Autodesk Inventor part; units mm, degrees
ref_plane "YZ Plane" through (0, 0, 0) normal (1, 0, 0) x (0, 1, 0)
ref_plane "XZ Plane" through (0, 0, 0) normal (0, 1, 0) x (-1, 0, 0)
ref_plane "XY Plane" through (0, 0, 0) normal (0, 0, 1) x (1, 0, 0)
sketch "Sketch1" plane through (0, 0, 0) normal (0, 1, 0) x (-1, 0, 0)
  line L0 (0, 0) -> (-10.25, 0)
  line L1 (-10.25, 0) -> (-10.25, -60)
  line L2 (-14.25, 4) -> (0, 4)
  line L3 (0, 4) -> (0, 0)
  line L4 (-10.25, -60) -> (-30.25, -60)
  line L5 (-30.25, -60) -> (-30.25, -56)
  line L6 (-30.25, -56) -> (-14.25, -56)
  line L7 (-14.25, -56) -> (-14.25, 4)
  dimension "d0" = 10.25
  dimension "d1" = 60
  dimension "d3" = 4
  dimension "d4" = 20
  dimension "d5" = 4
  dimension "d6" = 4
extrude "Extrusion1" add sketch "Sketch1" along normal blind 15
sketch "Sketch2" plane through (14.25, 0, -56) normal (0, 0, 1) x (1, 0, 0)
  line L0 (0, 15) -> (16, 0) construction
  line L1 (0, 0) -> (16, 15) construction
  point P0 (-14.25, 0)
  point P1 (8, 7.5)
hole "Hole1" at (22.25, 7.5, -56) direction (0, 0, -1) diameter 3.5 depth 8 tip angle 118
mirror "Mirror1" about plane through (0, 0, 0) normal (-1, 0, 0)
properties part number "clip" material "ABS Plastic"
Input: part model. Units: mm. Frame: model coordinates. A direction names the side the tool comes from. Round coordinates to 2 decimals unless told otherwise and drop trailing zeros. Loops run counter-clockwise (first coordinate to the right, second up) from the corner with the lowest first, then second, coordinate; pieces in that order, holes last. Notation, with made-up numbers: (35.25, 44.25) -> (69.25, 44.25) arc R8 ccw to (69.25, 54.25) -> close; hole circle Ø1 at (48.5, 26.25). An arc over 180 degrees is marked (long way). Write each question's results on one line, items separated by ' | '.
1. Ray query, line 1 (X direction, y = 7.5, z = -59.1); line 2 (X direction, y = 13, z = -21); line 3 (Y direction, x = -22, z = -58). Return the intervals inside material, ascending. Write a range as from..to.
Geometry results:
line 1: -30.25..-24, -20.5..-10.25, 10.25..20.5, 24..30.25 | line 2: -14.25..-10.25, 10.25..14.25 | line 3: 0..5.77, 9.23..15
2. Section B-B (y = 7.5). Return loops of the section in (x, z), and give its area (3 significant figures).
Geometry results:
outline: (-30.25, -60) -> (-24, -60) -> (-24, -56) -> (-30.25, -56) -> close; (-20.5, -60) -> (-10.25, -60) -> (-10.25, 0) -> (10.25, 0) -> (10.25, -60) -> (20.5, -60) -> (20.5, -56) -> (14.25, -56) -> (14.25, 4) -> (-14.25, 4) -> (-14.25, -56) -> (-20.5, -56) -> close; (24, -60) -> (30.25, -60) -> (30.25, -56) -> (24, -56) -> close | area: 694 mm2
3. First-contact query: P1, Ø5, axis at y = 11, z = -36.5, coming from the +X side; P2, Ø8, axis at x = -21.5, z = -44.5, coming from the -Y side; P3, Ø4.5, axis at y = 4, z = -18, coming from the -X side; P4, Ø5.5, axis at x = 22.25, y = 7.5, coming from the +Z side. Flat tips, straight axial feed; report the tip coordinate or a pass-through.
Geometry results:
P1: x = 14.25 | P2: through | P3: x = -14.25 | P4: z = -56
4. Section D-D (y = 12.5). Return loops of the section in (x, z), and give its area (3 significant figures).
Geometry results:
outline: (-30.25, -60) -> (-10.25, -60) -> (-10.25, 0) -> (10.25, 0) -> (10.25, -60) -> (30.25, -60) -> (30.25, -56) -> (14.25, -56) -> (14.25, 4) -> (-14.25, 4) -> (-14.25, -56) -> (-30.25, -56) -> close | area: 722 mm2
5. Section A-A (z = -51.5). Return loops of the section in (x, y), and give its area (3 significant figures).
Geometry results:
outline: (-14.25, 0) -> (-10.25, 0) -> (-10.25, 15) -> (-14.25, 15) -> close; (10.25, 0) -> (14.25, 0) -> (14.25, 15) -> (10.25, 15) -> close | area: 120 mm2
6. Mould query, pull axis X, two halves, no side actions, for faces 1 (the face through (10.25, 7, -30)), 2 (the face through (20, 7, -60)), 3 (the face through (-14.25, 7, -26)). Classes: +X half, -X half, draft (parallel to the pull), parting line (faces both ways), or undercut.
Geometry results:
face 1: undercut | face 2: draft | face 3: -X half
7. Section C-C (x = -22.25). Return loops of the section in (y, z), and give its area (3 significant figures).
Geometry results:
outline: (0, -60) -> (5.75, -60) -> (5.75, -56) -> (0, -56) -> close; (9.25, -60) -> (15, -60) -> (15, -56) -> (9.25, -56) -> close | area: 46.0 mm2
8. Set-up query: faces 4 (the face through (-20, 7, -56)), 5 (the face through (11, 15, -30)), 6 (the face through (0, 7, 0)), 7 (the face through (14.25, 7, -26)). Return all of +Z, -Z, +X, -X, +Y, -Y with unobstructed straight access to the full face (end or side cutting, diameter ignored); none if empty.
Geometry results:
face 4: +Z, -X, +Y, -Y | face 5: +Z, -Z, +X, -X, +Y | face 6: -Z, +Y, -Y | face 7: +Z, +X, +Y, -Y
